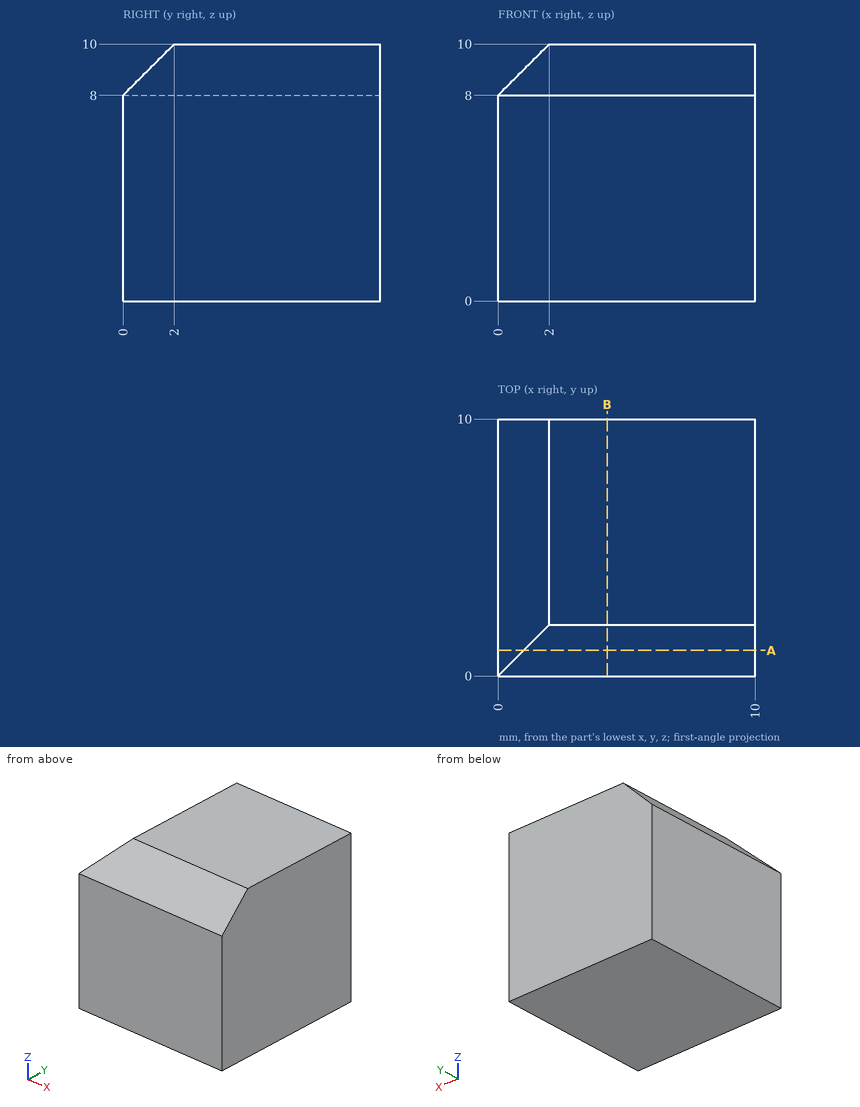
Check sheet for the drawn part. Datum: minimum x, y, z corner. Units: mm. Coordinates: 2 decimals unless noted, no trailing zeros. Loops run counter-clockwise (first coordinate to the right, second up) from the corner with the lowest first, then second, coordinate; pieces in that order, holes last. Notation, with made-up numbers: (3.25, 44.25) -> (44.25, 44.25) arc R16 ccw to (44.25, 53.25) -> close; hole circle Ø11 at (44, 61.25). An arc over 180 degrees is marked (long way). Answer as a JSON object with one key per item and string values. Group by question number.
Item 1: Sectioned sample at B-B on x = 4.25. Record the boundary of the cut face in (y, z), plus the area to 3 significant figures.
Item 2: Scan lines: probe 1 along Z at (x, y) = (2.75, 1); probe 2 along Z at (x, y) = (2, 1.25); probe 3 along X at (y, z) = (1.5, 9). Record each from-to range of solid material in increasing order.
Item 3: Sectioned sample at A-A on y = 1. Record the boundary of the cut face in (x, z).
Evaluation:
{
 "1": {"outline": "(0, 0) -> (10, 0) -> (10, 10) -> (2, 10) -> (0, 8) -> close", "area": "98.0 mm²"},
 "2": {"probe 1": "z = 0 to 9", "probe 2": "z = 0 to 9.25", "probe 3": "x = 1 to 10"},
 "3": {"outline": "(0, 0) -> (10, 0) -> (10, 9) -> (1, 9) -> (0, 8) -> close"}
}
